Model file for the job. Use its own axes, mm. A direction names the side the tool comes from. Round coordinates to 2 decimals unless told otherwise and drop trailing zeros. Loops run counter-clockwise (first coordinate to the right, second up) from the corner with the lowest first, then second, coordinate; pieces in that order, holes last. Notation, with made-up numbers: M 0.5,80.25 L 31.5,80.25 A12 cw 31.5,103.25 Z; hole C -7.5,3.25 d6. An arc over 180 degrees is marked long. Answer in a Markdown table with one row per item.
from build123d import *

# Parameters (mm, degrees)
BOSS_EXTRUDE1_DEPTH     = 3.175
CUT_EXTRUDE2_DEPTH      = 155.830786667
CUT_EXTRUDE2_DEPTH_BACK = 155.830786667
SKETCH3_R               = 1.25
SKETCH4_R               = 2.25
CUT_EXTRUDE3_DEPTH      = 155.830786667
CUT_EXTRUDE4_DEPTH      = 155.830786667
FILLET1_R               = 7


with BuildPart() as part:
    # Sketch1 → Boss-Extrude1 (new, symmetric)
    with BuildSketch(Plane.XY):
        with BuildLine():
            Line((92.5, 124), (-92.5, 124))
            Line((-92.5, 124), (-92.5, 94))
            Line((-92.5, 94), (-42.515070642, -18.833979089))
            ThreePointArc((-42.515070642, -18.833979089), (0, -46.5), (42.515070642, -18.833979089))
            Line((42.515070642, -18.833979089), (92.5, 94))
            Line((92.5, 94), (92.5, 124))
        make_face()
    extrude(amount=BOSS_EXTRUDE1_DEPTH, both=True)

    # Sketch3 → Cut-Extrude2 (cut, two sides: drawn at the far end of the back side and taken through both)
    with BuildSketch(Plane(origin=(0, 0, -3.175), x_dir=(-1, 0, 0), z_dir=(0, 0, -1)).offset(-CUT_EXTRUDE2_DEPTH_BACK)):
        with Locations((17.440159599, -16.121517706)):
            Circle(SKETCH3_R)
        with Locations((22.282044228, -8.220280106)):
            Circle(SKETCH3_R)
        with Locations((9.943168767, -21.568400378)):
            Circle(SKETCH3_R)
        with Locations((0.932420624, -23.731689611)):
            Circle(SKETCH3_R)
        with Locations((-8.220280106, -22.282044228)):
            Circle(SKETCH3_R)
        with Locations((-16.121517706, -17.440159599)):
            Circle(SKETCH3_R)
        with Locations((-21.568400378, -9.943168767)):
            Circle(SKETCH3_R)
        with Locations((-23.731689611, -0.932420624)):
            Circle(SKETCH3_R)
        with Locations((-22.282044228, 8.220280106)):
            Circle(SKETCH3_R)
        with Locations((-17.440159599, 16.121517706)):
            Circle(SKETCH3_R)
        with Locations((-9.943168767, 21.568400378)):
            Circle(SKETCH3_R)
        with Locations((-0.932420624, 23.731689611)):
            Circle(SKETCH3_R)
        with Locations((8.220280106, 22.282044228)):
            Circle(SKETCH3_R)
        with Locations((16.121517706, 17.440159599)):
            Circle(SKETCH3_R)
        with Locations((21.568400378, 9.943168767)):
            Circle(SKETCH3_R)
        with Locations((23.731689611, 0.932420624)):
            Circle(SKETCH3_R)
    extrude(amount=CUT_EXTRUDE2_DEPTH + CUT_EXTRUDE2_DEPTH_BACK, mode=Mode.SUBTRACT)

    # Sketch4 → Cut-Extrude3 (cut, through all)
    with BuildSketch(Plane(origin=(0, 0, -3.175), x_dir=(-1, 0, 0), z_dir=(0, 0, -1))):
        with Locations((67.5, 101.5)):
            Circle(SKETCH4_R)
        with Locations((87.5, 101.5)):
            Circle(SKETCH4_R)
        with Locations(Location((-87.5, 101.5, 0), (0, 0, 180))):
            Circle(SKETCH4_R)
        with Locations(Location((-67.5, 101.5, 0), (0, 0, 180))):
            Circle(SKETCH4_R)
        with Locations((-10, 101.5)):
            Circle(SKETCH4_R)
        with Locations((10, 101.5)):
            Circle(SKETCH4_R)
    extrude(amount=-CUT_EXTRUDE3_DEPTH, mode=Mode.SUBTRACT)

    # Sketch5 → Cut-Extrude4 (cut, through all)
    with BuildSketch(Plane(origin=(0, 0, -3.175), x_dir=(-1, 0, 0), z_dir=(0, 0, -1))):
        with BuildLine():
            Line((-15, 94), (-59.688105795, 94))
            Line((-59.688105795, 94), (-27.587967337, 21.538432121))
            ThreePointArc((-27.587967337, 21.538432121), (-21.882806981, 27.315613825), (-15, 31.622776602))
            Line((-15, 31.622776602), (-15, 94))
        make_face()
        with BuildLine():
            Line((59.688105795, 94), (27.587967337, 21.538432121))
            ThreePointArc((27.587967337, 21.538432121), (21.882806981, 27.315613825), (15, 31.622776602))
            Line((15, 31.622776602), (15, 94))
            Line((15, 94), (59.688105795, 94))
        make_face()
    extrude(amount=-CUT_EXTRUDE4_DEPTH, mode=Mode.SUBTRACT)

    # Fillet1
    fillet1_edges = [part.edges().sort_by_distance(p)[0] for p in [
        (15, 94, 0),
        (15, 31.622776602, 0),
        (27.587967337, 21.538432121, 0),
        (59.688105795, 94, 0),
        (-15, 94, 0),
        (-59.688105795, 94, 0),
        (-27.587967337, 21.538432121, 0),
        (-15, 31.622776602, 0),
    ]]
    fillet(fillet1_edges, radius=FILLET1_R)


solid = part.part
1. Wall check: probe 1 along X at (y, z) = (29, -2); probe 2 along X at (y, z) = (22, -2.5); probe 3 along Y at (x, z) = (-8.5, 1.5). Give the ranges that are in metal, low to high.
Verdict:
| item | result |
|---|---|
| probe 1 | x = -63.71 to -30.57, -19.6 to 19.6, 30.57 to 63.71 |
| probe 2 | x = -60.6 to -9.44, -7 to 8.77, 11.12 to 60.6 |
| probe 3 | y = -45.72 to 21.06, 23.5 to 99.82, 103.18 to 124 |
2. Mould opens along X. For faces 1 (the cylindrical face through (-89.58, 100.64, -0.04)), 2 (the cylindrical face through (17, 91.9, 0)), 3 (the flat face through (-1, 59, -3.175)), 4 (the flat face through (92.5, 109, 0)) say: +X half, -X half, draft (parallel to the pull), parting line (faces both ways), or undercut.
Verdict:
| item | result |
|---|---|
| face 1 | undercut |
| face 2 | undercut |
| face 3 | draft |
| face 4 | +X half |
3. Saw through at A-A (y = 101.5). Write the cut outline in (x, z) (3 decimals).
Verdict:
| item | result |
|---|---|
| outline | M -92.5,-3.175 L -89.75,-3.175 L -89.75,3.175 L -92.5,3.175 Z; M -85.25,-3.175 L -69.75,-3.175 L -69.75,3.175 L -85.25,3.175 Z; M -65.25,-3.175 L -12.25,-3.175 L -12.25,3.175 L -65.25,3.175 Z; M -7.75,-3.175 L 7.75,-3.175 L 7.75,3.175 L -7.75,3.175 Z; M 12.25,-3.175 L 65.25,-3.175 L 65.25,3.175 L 12.25,3.175 Z; M 69.75,-3.175 L 85.25,-3.175 L 85.25,3.175 L 69.75,3.175 Z; M 89.75,-3.175 L 92.5,-3.175 L 92.5,3.175 L 89.75,3.175 Z |
4. Tool access for faces 5 (the flat face through (15, 61, 0)), 6 (the flat face through (-67.857, 38.373, 0.044)): list every direction of +Z, -Z, +X, -X, +Y, -Y with a clear straight run to the whole face (end or side of a thin tool).
Verdict:
| item | result |
|---|---|
| face 5 | +Z, -Z |
| face 6 | +Z, -Z, -X, -Y |
5. Pin check, flat tips, straight feed: pin 1 (1.9 mm diameter, centred on x = 42, z = -0.5, fed in from -Y); pin 2 (3 mm diameter, centred on x = -16.12, y = 17.44, fed in from -Z) (3 decimals); pin 3 (2 mm diameter, centred on y = 52.5, z = -1.5, fed in from +X); pin 4 (3 mm diameter, centred on y = 84.5, z = 1.5, fed in from -X). Stop position of each tip, or through.
Verdict:
| item | result |
|---|---|
| pin 1 | stops at y = -21.84 |
| pin 2 | stops at z = -3.175 |
| pin 3 | stops at x = 74.56 |
| pin 4 | stops at x = -88.96 |
6. Saw through at D-D (z = 1.25). State how many separate pieces and enclosed holes the cut face has, and give its area (3 significant figures).
Verdict:
| item | result |
|---|---|
| separate pieces | 1 |
| enclosed holes | 24 |
| area | 18,400 mm² |
7. Saw through at B-B (x = 45). Write the cut outline in (y, z) (3 decimals).
Verdict:
| item | result |
|---|---|
| outline | M -13.225,-3.175 L 60.844,-3.175 L 60.844,3.175 L -13.225,3.175 Z; M 94,-3.175 L 124,-3.175 L 124,3.175 L 94,3.175 Z |
8. Saw through at C-C (y = 48). Write the cut outline in (x, z) (3 decimals), and give its area (3 significant figures).
Verdict:
| item | result |
|---|---|
| outline | M -72.122,-3.175 L -39.31,-3.175 L -39.31,3.175 L -72.122,3.175 Z; M -15,-3.175 L 15,-3.175 L 15,3.175 L -15,3.175 Z; M 39.31,-3.175 L 72.122,-3.175 L 72.122,3.175 L 39.31,3.175 Z |
| area | 607 mm² |
